Part model, mm, in its own coordinate system. A direction names the side the tool comes from. Give positions to 0.01 mm unless a question says otherwise; leave off trailing zeros. Order: outer loops, then holes, each group sorted by start corner. A loop starts at its lowest first (then second) coordinate and runs counter-clockwise, first axis right, second up.
1. Which spindle directions (+Z, -Z, +X, -X, +Y, -Y) get a long thin tool onto all of the face, cutting with end or side? Do faces 1 (the cylindrical face through (10, 3.1, -3.2)), 2 (the cylindrical face through (4, -2, 0)), 3 (the flat face through (-2, -1.5, 0)). Say none if no direction does.
2. Drop flat-ended pins along their axis: pin 1 Ø1 at (x, z) = (-9, -0.5) entering from +Y; pin 2 Ø1.2 at (y, z) = (-4, 0.5) entering from -X; pin 3 Ø5 at (x, y) = (2.5, -3) entering from -Z. Give the stop position or say it passes through.
3. Slice it at A-A on y = -2.5. List the corners of the cut face in (x, z), and give its area (3 significant figures).
4. Mould opens along Z. For faces 4 (the conical face through (-6.554, 2.233, 5.025)), 5 (the flat face through (-3, 0, -3)), 6 (the cylindrical face through (-11.99, 0.37, 0.53)) say: +Z half, -Z half, draft (parallel to the pull), parting line (faces both ways), or undercut.
5. Probe line 1 (Z direction, x = 0, y = 2.85); line 2 (Y direction, x = 9, z = -6.75). List the from-to ranges inside material, lowest first.
Autodesk Inventor part; units mm, degrees
ref_plane "YZ Plane" through (0, 0, 0) normal (1, 0, 0) x (0, 1, 0)
ref_plane "XZ Plane" through (0, 0, 0) normal (0, 1, 0) x (-1, 0, 0)
ref_plane "XY Plane" through (0, 0, 0) normal (0, 0, 1) x (1, 0, 0)
sketch "Sketch1" plane through (0, 0, 0) normal (0, 1, 0) x (-1, 0, 0)
  circle A0 centre (0, 0) radius 4
  line L0 (0, 0) -> (4, 0) construction
  line L1 (0, 0) -> (0, -4) construction
  line L2 (0, 0) -> (-4, 0) construction
  line L3 (0, 0) -> (0, 4) construction
  dimension "d0" = 8
extrude "Extrusion1" add sketch "Sketch1" against normal blind 3.5
ref_plane "Work Plane1" through (0, 0, 0) normal (0, 0, 1) x (1, 0, 0)
sketch "Sketch2" plane through (0, 0, 0) normal (0, 0, 1) x (1, 0, 0)
  line L0 (-4, 0) -> (4, 0)
  line L1 (4, 0) -> (12, 0)
  line L2 (14, 0.75) -> (14, 3)
  line L3 (12.5, 3.75) -> (10.5, 3.75)
  line L4 (0, 0) -> (0, 1.25)
  line L5 (4, 0) -> (4, 1.5959) construction
  line L6 (14, 0.75) -> (12, 0.75)
  line L7 (12, 0.75) -> (12, 0)
  line L8 (14, 3) -> (12.5, 3.75)
  line L9 (10.5, 2.5) -> (10.5, 3.75)
  line L10 (5.8611, 1.9477) -> (6, 1.8384)
  line L11 (6, 1.8384) -> (6.1093, 1.9773)
  line L12 (4.1093, 1.7392) -> (4, 1.6003)
  line L13 (4, 1.6003) -> (3.8611, 1.7097)
  line L14 (1.8611, 1.4716) -> (2, 1.3622)
  line L15 (2, 1.3622) -> (2.1093, 1.5011)
  line L16 (0, 1.25) -> (1.8611, 1.4716)
  line L17 (2.1093, 1.5011) -> (3.8611, 1.7097)
  line L18 (4.1093, 1.7392) -> (5.8611, 1.9477)
  line L19 (4, 1.6003) -> (4, 3.125) construction
  line L20 (6, 1.8384) -> (6, 3.125) construction
  line L21 (10.5, 3.125) -> (6, 3.125) construction
  line L22 (6, 3.125) -> (4, 3.125) construction
  line L23 (4, 3.125) -> (2, 3.125) construction
  line L24 (2, 3.125) -> (0, 3.125) construction
  line L25 (1.8611, 1.4716) -> (2.1093, 1.5011) construction
  line L26 (3.8611, 1.7097) -> (4.1093, 1.7392) construction
  line L27 (5.8611, 1.9477) -> (6.1093, 1.9773) construction
  line L28 (1.9852, 1.4863) -> (2, 1.3622) construction
  line L29 (4, 1.7262) -> (4, 1.6003) construction
  line L30 (2, 1.3622) -> (2, 3.125) construction
  line L31 (7.8611, 2.1858) -> (8, 2.0765)
  line L32 (8, 2.0765) -> (8.1093, 2.2154)
  line L33 (8, 2.0765) -> (8, 3.125) construction
  line L34 (6.1093, 1.9773) -> (7.8611, 2.1858)
  line L35 (8.1093, 2.2154) -> (10.5, 2.5)
  point P0 (6, 1.9643)
  dimension "d8" = 14
  dimension "d11" = 12
  dimension "d12" = 0.75
  dimension "d13" = 3
  dimension "d14" = 0.75
  dimension "d15" = 1.5
  dimension "d16" = 1.25
  dimension "d19" = 3.5
  dimension "d23" = 1.25
  dimension "d24" = 2
  dimension "d25" = 0.125
  dimension "d26" = 2
  dimension "d27" = 2
revolve "Revolution1" add sketch "Sketch2" angle 360 about axis through (0, 0, 0) along (0, 1, 0)
sketch "Sketch3" plane through (0, -3.5, 0) normal (0, -1, 0) x (1, 0, 0)
  point P0 (0, 0)
  point P1 (0, 0)
sketch "Sketch4" plane through (0, -3.5, 0) normal (0, -1, 0) x (1, 0, 0)
  circle A0 centre (0, 0) radius 4
  circle A1 centre (0, 0) radius 4
  arc A2 (0, -4) -> (0, 4) centre (0, 0) ccw
  line L0 (0, 4) -> (0, -4)
extrude "Extrusion2" add sketch "Sketch4" along normal blind 2 contours A0 L0 picked at (0.5785, 1.2013)
sketch "Sketch5" plane through (0, -3.5, 0) normal (0, -1, 0) x (1, 0, 0)
  line L0 (0, -4) -> (0, 4)
  arc A0 (0, 4) -> (0, -4) centre (0, 0) ccw
extrude "Extrusion3" cut sketch "Sketch5" against normal blind 2
properties part number "Caps 8mm Square Rounded Caps Male"
Data:
1. face 1: +Y
1. face 2: -Y
1. face 3: +Z, -Z, -X, -Y
2. pin 1: stops at y = 2.38
2. pin 2: stops at x = 0
2. pin 3: stops at z = -4
3. outline: (0, -4) arc R4 ccw to (0, 4) - close
3. area: 25.1 mm2
4. face 4: undercut
4. face 5: draft
4. face 6: parting line
5. line 1: z = -14 to -10.5, 10.5 to 14
5. line 2: y = 0 to 3.75
